Input: part model. Units: mm. Frame: model coordinates. Face numbers are marked on the shaded views. A direction names the side the tool comes from. Round coordinates to 2 decimals unless told otherwise and drop trailing zeros. Write each loop counter-clockwise with the first axis right and the second up, starting at its lowest first coordinate (ties: lowest second). Pieces come first, ordered by that corner, then holes. Notation, with made-up numbers: (43, -14.75) -> (92, -14.75) arc R32 cw to (92, 20.25) -> close; hole circle Ø3 at (82, 40.5). An arc over 180 degrees is marked (long way). Write item = value, one per line. Start each with the question number.
Autodesk Inventor part; units mm, degrees
ref_plane "YZ Plane" through (0, 0, 0) normal (1, 0, 0) x (0, 1, 0)
ref_plane "XZ Plane" through (0, 0, 0) normal (0, 1, 0) x (-1, 0, 0)
ref_plane "XY Plane" through (0, 0, 0) normal (0, 0, 1) x (1, 0, 0)
sketch "Sketch1" plane through (0, 0, 0) normal (0, 1, 0) x (-1, 0, 0)
  line L0 (4.8641, 4.8641) -> (-4.8641, 4.8641)
  line L1 (-4.8641, 4.8641) -> (-4.8641, -4.8641)
  line L2 (-4.8641, -4.8641) -> (4.8641, -4.8641)
  line L3 (4.8641, -4.8641) -> (4.8641, 4.8641)
  point P0 (0, 0)
  point P1 (4.8641, 0)
  point P2 (0, -4.8641)
  dimension "d0" = 9.7282
  dimension "d1" = 9.7282
extrude "Extrusion1" add sketch "Sketch1" along normal blind 1.0668
sketch "Sketch2" plane through (0, 1.0668, 0) normal (0, 1, 0) x (1, 0, 0)
  line L0 (-4.8641, -4.8641) -> (4.8641, -4.8641)
  line L1 (3.4798, -0.9779) -> (4.8641, -0.9779)
  line L2 (4.8641, -0.9779) -> (4.8641, 0.9779)
  line L3 (4.8641, 0.9779) -> (3.4798, 0.9779)
  line L4 (2.5019, 0) -> (2.5019, 0)
  arc A0 (2.5019, 0) -> (3.4798, -0.9779) centre (3.4798, 0) ccw
  arc A1 (3.4798, 0.9779) -> (2.5019, 0) centre (3.4798, 0) ccw
  line L5 (4.8641, -4.8641) -> (4.8641, 4.8641)
  line L6 (0, 2.5019) -> (0, 2.5019)
  line L7 (-0.9779, 3.4798) -> (-0.9779, 4.8641)
  line L8 (-0.9779, 4.8641) -> (0.9779, 4.8641)
  line L9 (0.9779, 4.8641) -> (0.9779, 3.4798)
  arc A2 (0, 2.5019) -> (0.9779, 3.4798) centre (0, 3.4798) ccw
  arc A3 (-0.9779, 3.4798) -> (0, 2.5019) centre (0, 3.4798) ccw
  line L10 (4.8641, 4.8641) -> (-4.8641, 4.8641)
  line L11 (-4.8641, -0.9779) -> (-3.4798, -0.9779)
  line L12 (-2.5019, 0) -> (-2.5019, 0)
  line L13 (-3.4798, 0.9779) -> (-4.8641, 0.9779)
  line L14 (-4.8641, 0.9779) -> (-4.8641, -0.9779)
  line L15 (-4.8641, 4.8641) -> (-4.8641, -4.8641)
  arc A4 (-3.4798, -0.9779) -> (-2.5019, 0) centre (-3.4798, 0) ccw
  arc A5 (-2.5019, 0) -> (-3.4798, 0.9779) centre (-3.4798, 0) ccw
  line L16 (-0.9779, -4.8641) -> (0.9779, -4.8641)
  line L17 (0.9779, -4.8641) -> (0.9779, -3.4798)
  line L18 (0, -2.5019) -> (0, -2.5019)
  line L19 (-0.9779, -3.4798) -> (-0.9779, -4.8641)
  arc A6 (0, -2.5019) -> (-0.9779, -3.4798) centre (0, -3.4798) ccw
  arc A7 (0.9779, -3.4798) -> (0, -2.5019) centre (0, -3.4798) ccw
  point P0 (0, 0)
  point P1 (4.8641, 0)
  point P2 (4.8641, 0)
  point P3 (0, -4.8641)
  point P4 (0, -4.8641)
  point P5 (0, -4.8641)
  point P6 (-0.9779, 2.5019)
  point P7 (0, 4.8641)
  point P8 (0, 4.8641)
  point P9 (-2.5019, 0.9779)
  point P10 (-4.8641, 0)
  point P11 (-4.8641, 0)
  point P12 (0.9779, -2.5019)
  point P13 (0, -4.8641)
  point P14 (0, -4.8641)
  dimension "d10" = 0.9779
  dimension "d11" = 1.9558
  dimension "d12" = 2.3622
  dimension "d13" = 2.3622
  dimension "d14" = 0.9779
  dimension "d15" = 2.3622
  dimension "d16" = 0.9779
  dimension "d17" = 2.3622
  dimension "d18" = 0.9779
extrude "Extrusion2" cut sketch "Sketch2" against normal blind 0.2794 contours L19 A6 A7 L17 L0 | L14 L13 A5 A4 L11 | L1 A0 A1 L3 L2 | L8 L9 A2 A3 L7
fillet "Fillet1" radius 0.2794 12 edges at (0, 1.0668, 2.5019) (0.9779, 1.0668, 4.1719) (-0.9779, 1.0668, 4.1719) (-4.1719, 1.0668, 0.9779) (-4.1719, 1.0668, -0.9779) (-2.5019, 1.0668, 0) (-0.9779, 1.0668, -4.172) (0.9779, 1.0668, -4.172) (0, 1.0668, -2.5019) (4.172, 1.0668, -0.9779) (4.172, 1.0668, 0.9779) (2.5019, 1.0668, 0)
sketch "Sketch3" plane through (0, 1.0668, 0) normal (0, 1, 0) x (1, 0, 0)
  circle A0 centre (0, 0) radius 1.9685
  dimension "d22" = 3.937
extrude "Extrusion3" cut sketch "Sketch3" against normal through all
chamfer "Chamfer1" distance 0.0254 angle 45 16 edges at (3.0605, 1.0668, 4.8641) (1.0596, 0.9851, 4.8641) (4.8641, 1.0668, 3.0604) (4.8641, 0.9851, 1.0596) (4.8641, 1.0668, -3.0605) (4.8641, 0.9851, -1.0596) (3.0605, 1.0668, -4.8641) (1.0596, 0.9851, -4.8641) (-3.0605, 1.0668, -4.8641) (-1.0596, 0.9851, -4.8641) (-4.8641, 1.0668, -3.0605) (-4.8641, 0.9851, -1.0596) (-4.8641, 1.0668, 3.0605) (-4.8641, 0.9851, 1.0596) (-3.0605, 1.0668, 4.8641) (-1.0596, 0.9851, 4.8641)
chamfer "Chamfer2" distance 1.27 angle 45 4 edges at (4.8514, 1.0541, 4.8514) (4.8514, 1.0541, -4.8514) (-4.8514, 1.0541, -4.8514) (-4.8514, 1.0541, 4.8514)
properties part number "SSR-40 DA Small Plate" material "Nickel-Copper Alloy 400"
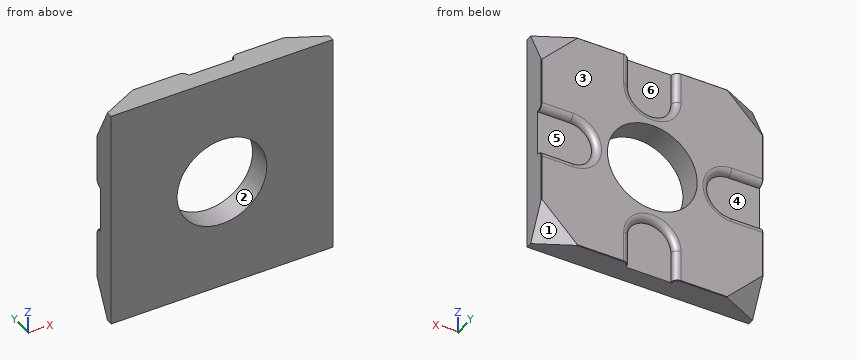
1. Reachability of the marked faces 4, 5 and 6 from +Z, -Z, +X, -X, +Y, -Y: full face, straight path, thin tool, end or side. Return the list, or none.
2. Line query: line 1 along Z through (x, y) = (0, 0.3); line 2 along Y through (x, z) = (4.75, 0). Output: solid intervals per line, ascending.
3. Section C-C (y = 0.45). Output: boundary loops of the cut face in (x, z), then the cut area to 3 significant figures.
4. Pin query (flat end, axial travel): P1, Ø0.6, axis at x = -0.5, z = -4, coming from the +Y side; P2, Ø4.5, axis at x = 0, z = 0, coming from the -Y side. Return the tip coordinate at first contact, or that it passes through.
5. Mould query, pull axis Z, two halves, no side actions, for the marked faces 1, 2 and 3. Classes: pulls with the +Z half, pulls with the -Z half, needs draft (parallel to the pull), parting line crosses it, or undercut.
Check sheet entries:
q1.face_4 = -X, +Y
q1.face_5 = +X, +Y
q1.face_6 = +Z, +Y
q2.line_1 = -4.86 to -1.97, 1.97 to 4.86
q2.line_2 = 0 to 0.79
q3.outline = (-4.86, -4.49) -> (-4.49, -4.86) -> (4.49, -4.86) -> (4.86, -4.49) -> (4.86, 4.49) -> (4.49, 4.86) -> (-4.49, 4.86) -> (-4.86, 4.49) -> close; hole circle Ø3.94 at (0, 0)
q3.area = 82.2 mm2
q4.P1 = 0.79
q4.P2 = 0
q5.face_1 = pulls with the -Z half
q5.face_2 = undercut
q5.face_3 = needs draft
